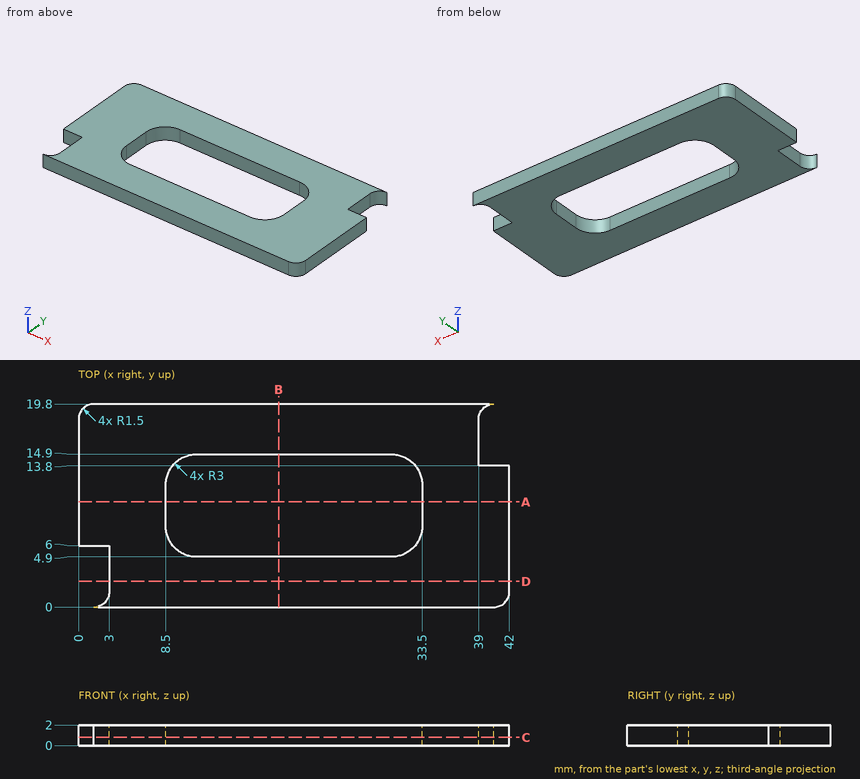
Job drawing, mm, ordinate dimensions from the low corner. One solid piece. Coordinates: 2 decimals unless noted, no trailing zeros. Write each loop counter-clockwise with the first axis right and the second up, starting at its lowest first coordinate (ties: lowest second). Pieces come first, ordered by that corner, then holes. Notation, with made-up numbers: M -10.5,1.5 L 47.5,1.5 A7 cw 47.5,14.5 Z; hole C -35,82 d11. An arc over 180 degrees is marked long. Answer as a JSON object with one key per item and string values. Group by question number.
1) Saw through at A-A (y = 10.25). Write the cut outline in (x, z).
2) Pin check, flat tips, straight feed: pin 1 Ø0.6 at (y, z) = (15, 1) entering from +X; pin 2 Ø0.6 at (x, z) = (41, 1) entering from +Y; pin 3 Ø1.5 at (x, y) = (31.5, 4) entering from -Z. Stop position of each tip, or through.
3) Saw through at D-D (y = 2.5). Write the cut outline in (x, z), plus the area to 3 significant figures.
4) Saw through at B-B (x = 19.5). Write the cut outline in (y, z).
5) Saw through at C-C (z = 0.8). Write the cut outline in (x, y), plus the area to 3 significant figures.
6) Wall check: line 1 (Y direction, x = 15.5, z = 1.2); line 2 (X direction, y = 8, z = 1.7); line 3 (X direction, y = 6.75, z = 0.3). Give the ranges that are in metal, low to high. Write a range as from..to.
Values follow:
{
 "1": {"outline": "M 0,0 L 8.5,0 L 8.5,2 L 0,2 Z; M 33.5,0 L 42,0 L 42,2 L 33.5,2 Z"},
 "2": {"pin 1": "stops at x = 39", "pin 2": "stops at y = 13.8", "pin 3": "stops at z = 0"},
 "3": {"outline": "M 3,0 L 42,0 L 42,2 L 3,2 Z", "area": "78.0 mm2"},
 "4": {"outline": "M 0,0 L 4.9,0 L 4.9,2 L 0,2 Z; M 14.9,0 L 19.8,0 L 19.8,2 L 14.9,2 Z"},
 "5": {"outline": "M 0,6 L 3,6 L 3,1.5 A1.5 cw 1.5,0 L 40.5,0 A1.5 ccw 42,1.5 L 42,13.8 L 39,13.8 L 39,18.3 A1.5 cw 40.5,19.8 L 1.5,19.8 A1.5 ccw 0,18.3 Z; hole M 8.5,7.9 A3 ccw 11.5,4.9 L 30.5,4.9 A3 ccw 33.5,7.9 L 33.5,11.9 A3 ccw 30.5,14.9 L 11.5,14.9 A3 ccw 8.5,11.9 Z", "area": "553 mm2"},
 "6": {"line 1": "y = 0..4.9, 14.9..19.8", "line 2": "x = 0..8.5, 33.5..42", "line 3": "x = 0..8.73, 33.27..42"}
}
